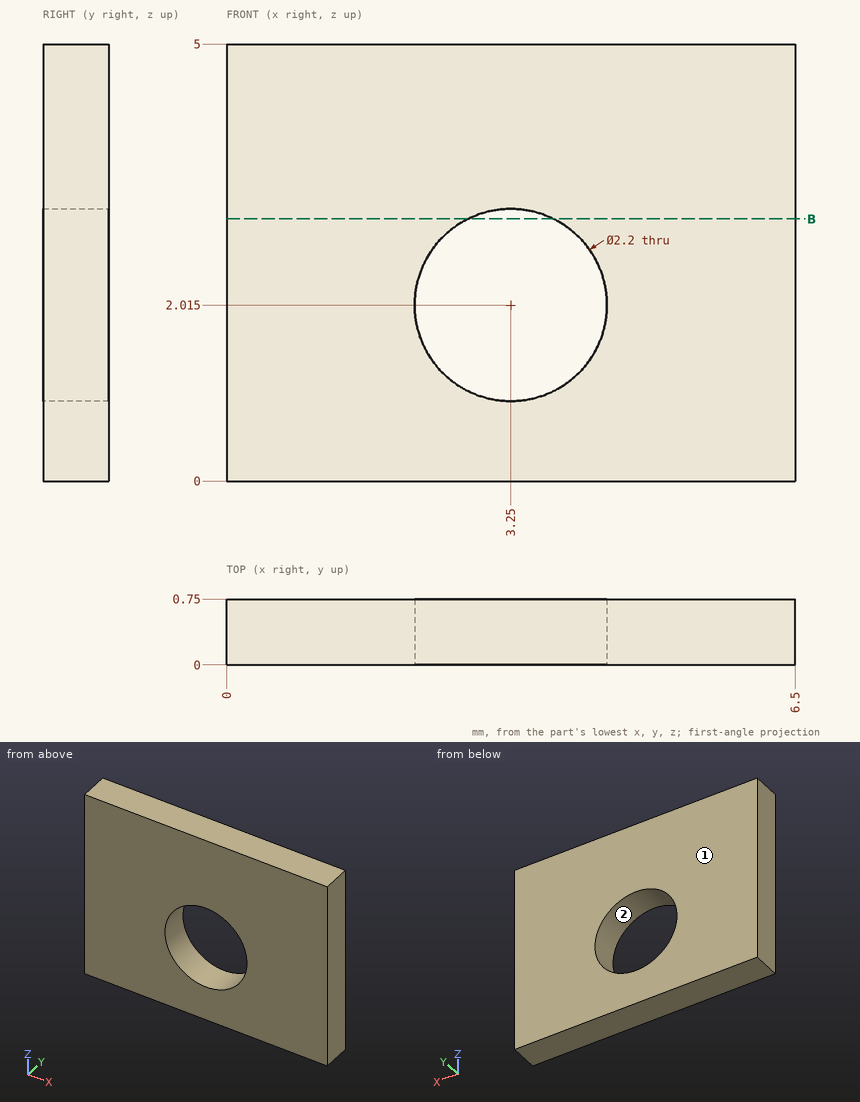
Here's the drawing with two shaded views (mm, measured from the low corner). I have some questions. Give positions to 0.01 mm unless a question says otherwise; leave off trailing zeros. Order: outer loops, then holes, each group sorted by start corner. A loop starts at its lowest first (then second) coordinate and runs counter-clockwise, first axis right, second up.
Q1. I'm going to push a flat-ended pin straight in: P1, Ø1.3, axis at x = 3.25, z = 2.02, coming from the -Y side. Where does the tip first touch, or does it pass through?
Q2. We'd pull the mould along Z, two halves only. Please class the marked faces 1 and 2: +Z half, -Z half, draft (parallel to the pull), parting line (faces both ways), or undercut.
Q3. If I drill on line 1 along Z through (x, y) = (3.25, 0.45) (1 decimal); line 2 along Z through (x, y) = (3.75, 0.25) (1 decimal); line 3 along X through (y, z) = (0.5, 1.65), over which ranges is the centre line in solid material (lowest first)?
Q4. Suppose I cut it at B-B, the plane z = 3. Write out the boundary of the cut face in (x, y).
Solution:
1. P1: passes through
2. face 1: draft
2. face 2: undercut
3. line 1: z = 0 to 0.9, 3.1 to 5
3. line 2: z = 0 to 1, 3 to 5
3. line 3: x = 0 to 2.21, 4.29 to 6.5
4. outline: (0, 0) - (2.76, 0) - (2.76, 0.75) - (0, 0.75) - close; (3.74, 0) - (6.5, 0) - (6.5, 0.75) - (3.74, 0.75) - close
